Build history of the part. All positions in model axes, mm. Face numbers are marked on the shaded views. A direction names the side the tool comes from. Give positions to 0.01 mm unless a question says otherwise; leave off trailing zeros. Write each loop counter-clockwise with the first axis right and the second up, starting at its lowest first coordinate (ties: lowest second). Pieces come first, ordered by that corner, then holes. Notation, with made-up numbers: (57, -34) -> (111, -34) arc R22 cw to (111, -22) -> close; hole circle Ø4 at (63.25, 45.25). An arc over 180 degrees is marked (long way). Write item = value, one per line. Start each with the question number.
Q1. Saw through at A-A, the plane y = 16.51. List the corners of the cut face in (x, z) (3 decimals).
Q2. Mould opens along X. For the marked faces 1, 2 and 3 say: pulls with the +X half, pulls with the -X half, needs draft (parallel to the pull), parting line crosses it, or undercut.
Q3. Tool access for the marked faces 4, 5, 6, 7 and 8: list every direction of +Z, -Z, +X, -X, +Y, -Y with a clear straight run to the whole face (end or side of a thin tool).
Q4. Saw through at D-D, the plane y = 3. List the corners of the cut face in (x, z).
Q5. Drop flat-ended pins along their axis: P1, Ø5.5, axis at x = -24.13, y = 16.51, coming from the +Z side; P2, Ø1.9, axis at y = -15, z = 4.5, coming from the +X side; P3, Ø11, axis at x = 9.525, y = -10.541, coming from the +Z side; P4, Ø6.5, axis at x = -9.525, y = -10.541, coming from the +Z side. Give the stop position or say it passes through.
Q6. Saw through at C-C, the plane z = 1.5. Give the number of separate pieces and of enclosed holes in the cut face, then the cut area to 3 significant figures.
Q7. Saw through at B-B, the plane x = -24.13. List the corners of the cut face in (y, z), then the cut area to 3 significant figures.
Q8. Wall check: line 1 (X direction, y = 6.35, z = 1.1) (3 decimals); line 2 (Y direction, x = 24.13, z = 2.7); line 3 (X direction, y = 5.5, z = 0.5) (3 decimals). Give the ranges that are in metal, low to high.
from build123d import *

# Parameters (mm, degrees)
SKETCH1_R           = 3.475
SKETCH1_R_2         = 2.3828
BOSS_EXTRUDE1_DEPTH = 6.35
CHAMFER1_SIZE       = 3
CHAMFER2_SIZE       = 8
CUT_EXTRUDE1_DEPTH  = 2.286
SKETCH4_W           = 40.986
SKETCH4_H           = 20.158
CUT_EXTRUDE2_DEPTH  = 36.817152344


with BuildPart() as part:
    # Sketch1 → Boss-Extrude1 (new body)
    with BuildSketch(Plane.XY):
        Polygon((17.4625, -21.209), (-17.4625, -21.209), (-17.4625, 1.651), (-28.575, 1.651), (-28.575, 21.209), (28.575, 21.209), (28.575, 1.651), (17.4625, 1.651), align=None)
        with Locations((-9.525, -10.541)):
            Circle(SKETCH1_R, mode=Mode.SUBTRACT)
        with Locations((9.525, -10.541)):
            Circle(SKETCH1_R, mode=Mode.SUBTRACT)
        with Locations((-24.13, 6.35)):
            Circle(SKETCH1_R_2, mode=Mode.SUBTRACT)
        with Locations((-24.13, 16.51)):
            Circle(SKETCH1_R_2, mode=Mode.SUBTRACT)
        with Locations((24.13, 16.51)):
            Circle(SKETCH1_R_2, mode=Mode.SUBTRACT)
        with Locations((24.13, 6.35)):
            Circle(SKETCH1_R_2, mode=Mode.SUBTRACT)
    extrude(amount=BOSS_EXTRUDE1_DEPTH)

    # Chamfer1
    chamfer1_edges = [part.edges().sort_by_distance(p)[0] for p in [
        (-28.575, 1.651, 3.175),
        (-28.575, 21.209, 3.175),
        (28.575, 21.209, 3.175),
        (28.575, 1.651, 3.175),
        (17.4625, -21.209, 3.175),
        (-17.4625, -21.209, 3.175),
    ]]
    chamfer(chamfer1_edges, length=CHAMFER1_SIZE)

    # Chamfer2
    chamfer2_edges = [part.edges().sort_by_distance(p)[0] for p in [
        (17.4625, 1.651, 3.175),
        (-17.4625, 1.651, 3.175),
    ]]
    chamfer(chamfer2_edges, length=CHAMFER2_SIZE)

    # Sketch3 → Cut-Extrude1 (cut)
    with BuildSketch(Plane.XY.offset(6.35)):
        Polygon((-25.4625, 1.651), (25.4625, 1.651), (25.575, 1.651), (28.575, 4.651), (28.575, 18.209), (25.575, 21.209), (-25.575, 21.209), (-28.575, 18.209), (-28.575, 4.651), (-25.575, 1.651), align=None)
    extrude(amount=-CUT_EXTRUDE1_DEPTH, mode=Mode.SUBTRACT)

    # Sketch4 → Cut-Extrude2 (cut, through all)
    with BuildSketch(Plane.XY.offset(4.064)):
        with Locations((0, 11.43)):
            Rectangle(SKETCH4_W, SKETCH4_H)
    extrude(amount=-CUT_EXTRUDE2_DEPTH, mode=Mode.SUBTRACT)


solid = part.part
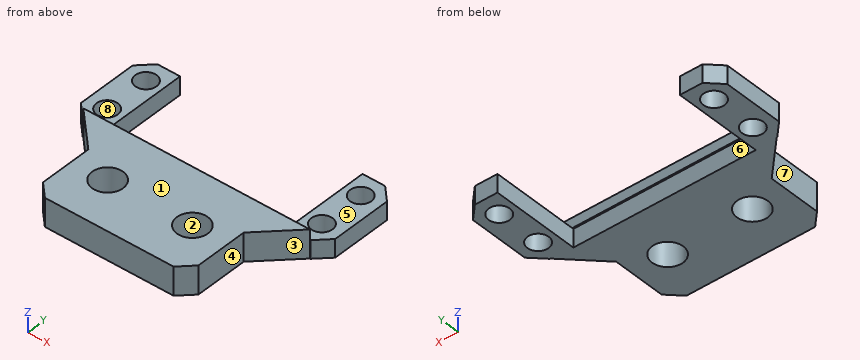
Report:
q1.outline = (-28.575, 0) -> (-26.513, 0) -> (-26.513, 4.064) -> (-28.575, 4.064) -> close; (-21.747, 0) -> (-20.493, 0) -> (-20.493, 4.064) -> (-21.747, 4.064) -> close; (20.493, 0) -> (21.747, 0) -> (21.747, 4.064) -> (20.493, 4.064) -> close; (26.513, 0) -> (28.575, 0) -> (28.575, 4.064) -> (26.513, 4.064) -> close
q2.face_1 = needs draft
q2.face_2 = undercut
q2.face_3 = pulls with the +X half
q3.face_4 = +Z, -Z, +X, -Y
q3.face_5 = +Z, +X, -X, +Y
q3.face_6 = -Z, +Y
q3.face_7 = +Z, -Z, -X, -Y
q3.face_8 = +Z, -Z
q4.outline = (-26.92, 0) -> (-20.49, 0) -> (-20.49, 4.06) -> (-26.92, 4.06) -> close; (20.49, 0) -> (26.92, 0) -> (26.92, 4.06) -> (20.49, 4.06) -> close
q5.P1 = 4.06
q5.P2 = 17.46
q5.P3 = 6.35
q5.P4 = through
q6.separate_pieces = 1
q6.enclosed_holes = 6
q6.area = 992 mm2
q7.outline = (0.32, 0) -> (3.97, 0) -> (3.97, 4.06) -> (1.65, 4.06) -> (1.65, 6.35) -> (0.32, 6.35) -> close; (8.73, 0) -> (14.13, 0) -> (14.13, 4.06) -> (8.73, 4.06) -> close; (18.89, 0) -> (21.21, 0) -> (21.21, 4.06) -> (18.89, 4.06) -> close
q7.area = 49.2 mm2
q8.line_1 = -28.575 to -26.513, -21.747 to -20.493, 20.493 to 21.747, 26.513 to 28.575
q8.line_2 = 0.32 to 3.97, 8.73 to 14.13, 18.89 to 21.21
q8.line_3 = -28.575 to -26.356, -21.904 to -20.493, 20.493 to 21.904, 26.356 to 28.575
